Input: dimensioned drawing with shaded views. Units: mm. Origin: part minimum x, y, z. A direction names the side the tool comes from. Give positions to 0.01 mm unless a question says otherwise; leave off trailing zeros. Write each loop counter-clockwise with the first axis right and the second up, starting at its lowest first coordinate (ties: lowest second). Pieces come first, ordered by that corner, then holes.
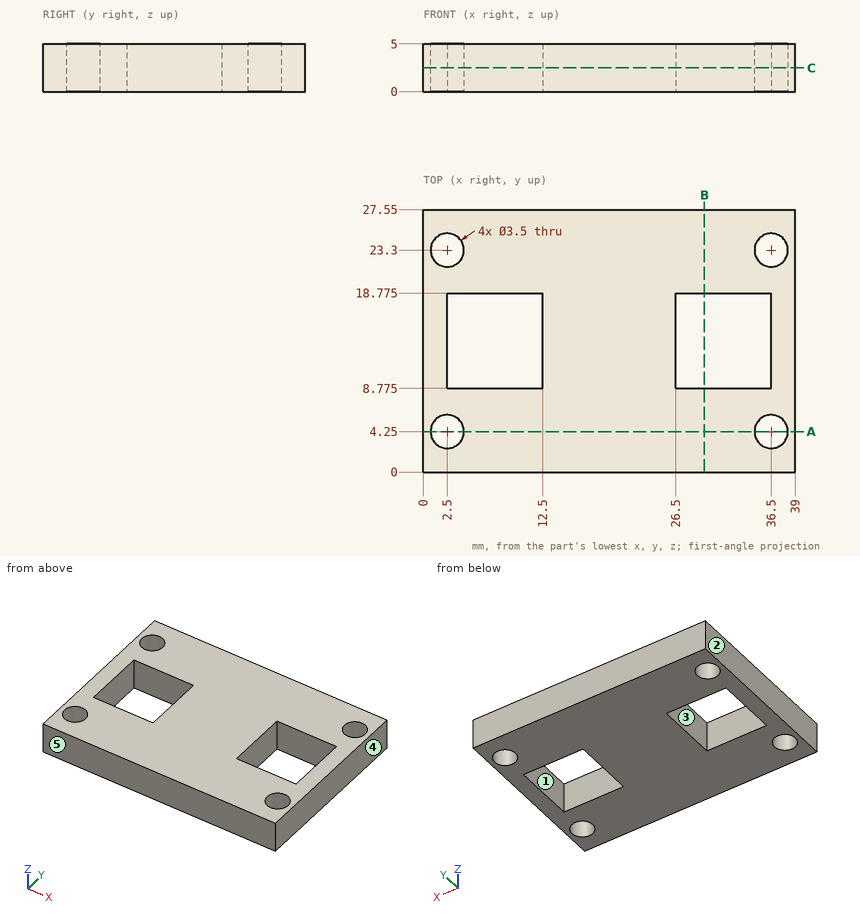
Item 1: Section A-A, the plane y = 4.25. Return the cut outline in (x, z).
Found:
outline: (0, 0) - (0.75, 0) - (0.75, 5) - (0, 5) - close; (4.25, 0) - (34.75, 0) - (34.75, 5) - (4.25, 5) - close; (38.25, 0) - (39, 0) - (39, 5) - (38.25, 5) - close
Item 2: Section C-C, the plane z = 2.5. Return the cut outline in (x, y) (3 decimals), plus the area to 3 significant figures.
Found:
outline: (0, 0) - (39, 0) - (39, 27.55) - (0, 27.55) - close; hole circle Ø3.5 at (2.5, 4.25); hole circle Ø3.5 at (2.5, 23.3); hole (2.5, 8.775) - (12.5, 8.775) - (12.5, 18.775) - (2.5, 18.775) - close; hole (26.5, 8.775) - (36.5, 8.775) - (36.5, 18.775) - (26.5, 18.775) - close; hole circle Ø3.5 at (36.5, 4.25); hole circle Ø3.5 at (36.5, 23.3)
area: 836 mm2
Item 3: Section B-B, the plane x = 29.5. Return the cut outline in (y, z) (3 decimals), plus the area to 4 significant figures.
Found:
outline: (0, 0) - (8.775, 0) - (8.775, 5) - (0, 5) - close; (18.775, 0) - (27.55, 0) - (27.55, 5) - (18.775, 5) - close
area: 87.75 mm2
Item 4: Pull-direction query (X, two-part tool) for the marked faces 3, 4 and 5; classes: +X half, -X half, draft (parallel to the pull), parting line (faces both ways), or undercut.
Found:
face 3: undercut
face 4: +X half
face 5: draft
Item 5: Line query: L1, parallel to X at y = 11.75, z = 2.05; L2, parallel to Y at x = 9, z = 0.95 (3 decimals); L3, parallel to X at y = 23, z = 3.7. Output: solid intervals per line, ascending.
Found:
L1: x = 0 to 2.5, 12.5 to 26.5, 36.5 to 39
L2: y = 0 to 8.775, 18.775 to 27.55
L3: x = 0 to 0.78, 4.22 to 34.78, 38.22 to 39
Item 6: Pin query (flat end, axial travel): pin 1 Ø4.5 at (x, y) = (36.5, 23.3) entering from -Z. Return the tip coordinate at first contact, or that it passes through.
Found:
pin 1: stops at z = 0
Item 7: Reachability of the marked faces 1 and 2 from +Z, -Z, +X, -X, +Y, -Y: full face, straight path, thin tool, end or side. Return the list, or none.
Found:
face 1: +Z, -Z
face 2: +Z, -Z, -X, +Y, -Y
